Can you work these out from the drawing? Everything is in mm from the part's minimum corner. Coordinates: 2 decimals unless noted, no trailing zeros. Loops run counter-clockwise (first coordinate to the right, second up) from the corner with the lowest first, then second, coordinate; pieces in that order, holes last.
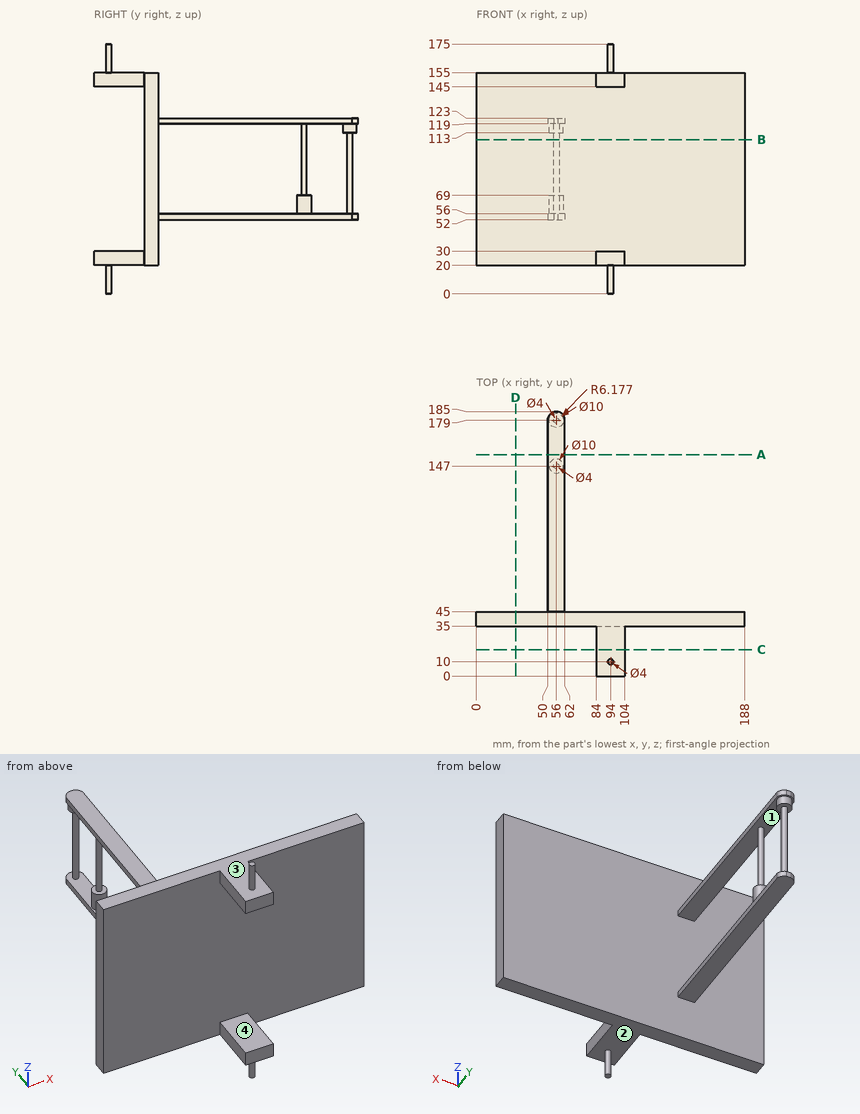
1) We'd pull the mould along Z, two halves only. Please class the marked faces 1, 2, 3 and 4: released by +Z, released by -Z, zero draft, split by the parting line, or undercut.
2) Imagine slicing it at B-B on z = 108. List the corners of the cut face in (x, y) for me.
3) Imagine slicing it at C-C on y = 18.5. List the corners of the cut face in (x, z) for me.
4) Will these pins go through, and if not, where does the flat tip stop? pin 1 (1.5 mm diameter, centred on x = 59, z = 49, fed in from +Y); pin 2 (8 mm diameter, centred on y = 14, z = 150, fed in from +X); pin 3 (5 mm diameter, centred on x = 57, y = 181.5, fed in from -Z).
5) Imagine slicing it at A-A on y = 155. List the corners of the cut face in (x, z) for me, plus the area to 3 significant figures.
6) If I drill on L1, parallel to Z at x = 55.5, y = 172; L2, parallel to Z at x = 86, y = 8; L3, parallel to Y at x = 12.5, z = 127, over which ranges is the centre line in solid material (lowest first)?
7) Imagine slicing it at D-D on x = 27.5. List the corners of the cut face in (y, z) for me, plus the area to 3 significant figures.
Solved:
1. face 1: undercut
1. face 2: released by -Z
1. face 3: released by +Z
1. face 4: undercut
2. outline: (0, 35) - (188, 35) - (188, 45) - (0, 45) - close; circle Ø4 at (56, 147); circle Ø4 at (56, 179)
3. outline: (84, 20) - (104, 20) - (104, 30) - (84, 30) - close; (84, 145) - (104, 145) - (104, 155) - (84, 155) - close
4. pin 1: stops at y = 45
4. pin 2: stops at x = 104
4. pin 3: stops at z = 52
5. outline: (50, 52) - (62, 52) - (62, 56) - (50, 56) - close; (50, 119) - (62, 119) - (62, 123) - (50, 123) - close
5. area: 96.0 mm2
6. L1: z = 52 to 56, 119 to 123
6. L2: z = 20 to 30, 145 to 155
6. L3: y = 35 to 45
7. outline: (35, 20) - (45, 20) - (45, 155) - (35, 155) - close
7. area: 1,350 mm2
